from build123d import *

# Parameters (mm, degrees)
SKETCH2_W           = 100
SKETCH2_H           = 100
SKETCH2_R           = 12.5
BOSS_EXTRUDE1_DEPTH = 3
SKETCH3_W           = 7
SKETCH3_H           = 7
BOSS_EXTRUDE2_DEPTH = 5
SKETCH4_W           = 3
SKETCH4_H           = 8
SKETCH4_W_2         = 8
SKETCH4_H_2         = 3
BOSS_EXTRUDE3_DEPTH = 7
SKETCH5_R           = 1.6
CUT_EXTRUDE1_DEPTH  = 111.308657865
SKETCH8_R           = 1.6
CUT_EXTRUDE4_DEPTH  = 111.308657865
SKETCH9_R           = 3
CUT_EXTRUDE5_DEPTH  = 10
FILLET1_R           = 0.5


with BuildPart() as part:
    # Sketch2 → Boss-Extrude1 (new body)
    with BuildSketch(Plane(origin=(0, 0, 0), x_dir=(1, 0, 0), z_dir=(0, 1, 0))):
        Rectangle(SKETCH2_W, SKETCH2_H)
        with Locations(Location((0, 0, 0), (0, 0, 270))):
            Circle(SKETCH2_R, mode=Mode.SUBTRACT)
    extrude(amount=BOSS_EXTRUDE1_DEPTH)

    # Sketch3 → Boss-Extrude2 (add)
    with BuildSketch(Plane(origin=(0, 3, 0), x_dir=(1, 0, 0), z_dir=(0, 1, 0))):
        with Locations((-46.5, 46.5)):
            Rectangle(SKETCH3_W, SKETCH3_H)
        with Locations((46.5, 46.5)):
            Rectangle(SKETCH3_W, SKETCH3_H)
        with Locations((46.5, -46.5)):
            Rectangle(SKETCH3_W, SKETCH3_H)
        with Locations((-46.5, -46.5)):
            Rectangle(SKETCH3_W, SKETCH3_H)
    extrude(amount=BOSS_EXTRUDE2_DEPTH)

    # Sketch4 → Boss-Extrude3 (add)
    with BuildSketch(Plane.XZ):
        with Locations((46.5, -39)):
            Rectangle(SKETCH4_W, SKETCH4_H)
        with Locations((39, 46.5)):
            Rectangle(SKETCH4_W_2, SKETCH4_H_2)
        with Locations((-46.5, 39)):
            Rectangle(SKETCH4_W, SKETCH4_H)
        with Locations((-39, -46.5)):
            Rectangle(SKETCH4_W_2, SKETCH4_H_2)
    extrude(amount=BOSS_EXTRUDE3_DEPTH)

    # Sketch5 → Cut-Extrude1 (cut, through all)
    with BuildSketch(Plane(origin=(0, 0, -48), x_dir=(-1, 0, 0), z_dir=(0, 0, -1))):
        with Locations((39, -3.5)):
            Circle(SKETCH5_R)
        with Locations((-39, -3.5)):
            Circle(SKETCH5_R)
    extrude(amount=-CUT_EXTRUDE1_DEPTH, mode=Mode.SUBTRACT)

    # Sketch8 → Cut-Extrude4 (cut, through all)
    with BuildSketch(Plane(origin=(48, 0, 0), x_dir=(0, 0, -1), z_dir=(1, 0, 0))):
        with Locations((-39, -3.5)):
            Circle(SKETCH8_R)
        with Locations((39, -3.5)):
            Circle(SKETCH8_R)
    extrude(amount=-CUT_EXTRUDE4_DEPTH, mode=Mode.SUBTRACT)

    # Sketch9 → Cut-Extrude5 (cut)
    with BuildSketch(Plane(origin=(0, 3, 0), x_dir=(1, 0, 0), z_dir=(0, 1, 0))):
        with Locations(Location((-27.876571837, 0, 0), (0, 0, 270))):
            Circle(SKETCH9_R)
    extrude(amount=-CUT_EXTRUDE5_DEPTH, mode=Mode.SUBTRACT)

    # Fillet1
    fillet1_edges = [part.edges().sort_by_distance(p)[0] for p in [
        (-50, 4, 50),
        (-50, 4, -50),
        (50, 4, -50),
        (50, 4, 50),
    ]]
    fillet(fillet1_edges, radius=FILLET1_R)


solid = part.part
Work out the finished part from the listing and answer in its coordinate system (mm). A direction names the side the tool comes from. Give positions to 0.01 mm unless a question says otherwise; leave off trailing zeros. Write each loop counter-clockwise with the first axis right and the second up, starting at its lowest first coordinate (ties: lowest second). Pieces come first, ordered by that corner, then holes. Notation, with made-up numbers: (70, -26) - (90, -26) arc R20 ccw to (90, -20) - close; hole circle Ø4 at (-35, 61). An arc over 180 degrees is marked (long way). One line per item, written item: value. Start each with the question number.
1. For faces 1 (the flat face through (46, -3, -43)), 2 (the flat face through (43, 5, 47)), 3 (the flat face through (-43, -3, -47)), 4 (the flat face through (38, -2, 48)), 5 (the flat face through (-35, -3, -47)), determine the directions among +Z, -Z, +X, -X, +Y, -Y from which every point of the face is accessible in a straight line to the end or side of a thin tool.
2. Find section B-B (y = -3.5). State how many separate pieces and enclosed holes the cut face has, then the cut area to 3 significant figures.
3. Given pin 1 (2 mm diameter, centred on y = -4.5, z = 39.5, fed in from -X); pin 2 (3.5 mm diameter, centred on y = -5, z = 46.5, fed in from +X); pin 3 (0.9 mm diameter, centred on x = 47, y = -4, fed in from -Z); pin 4 (2 mm diameter, centred on y = 5, z = 19.5, fed in from -X), each flat-ended and moving along its own axis, determine where each tip first touches the part or whether it passes through.
4. Consider probe 1 along X at (y, z) = (0.7, 0); probe 2 along Y at (x, z) = (46.25, -39); probe 3 along Y at (x, z) = (-19.5, 21). Determine where each line is inside the solid, lowest interval first.
5. Find section A-A (z = 39). Write down the section's boundary in (x, y), then the cut area to 3 significant figures.
6. Find section D-D (z = 10). Write down the section's boundary in (x, y).
7. For a pull along Z with two mould halves and no side action, classify faces 6 (the flat face through (45, -2, -40)), 7 (the cylindrical face through (46.521, -1.914, -38.792)), 8 (the cylindrical face through (-30.805, 1.521, -0.65)), 9 (the flat face through (38, -2, 45)) as +Z half, -Z half, draft (parallel to the pull), parting line (faces both ways), or undercut.
8. Find section C-C (x = 39). Write down the section's boundary in (y, z), then the cut area to 3 significant figures.
Geometry results:
1. face 1: -Z, +X, -X, -Y
1. face 2: +Z, -Z, +Y
1. face 3: +Z, -Z, -X, -Y
1. face 4: +Z, +X, -X, -Y
1. face 5: +Z, -Z, +X, -Y
2. separate pieces: 8
2. enclosed holes: 0
2. area: 57.6 mm2
3. pin 1: x = -48
3. pin 2: x = 43
3. pin 3: z = -43
3. pin 4: through
4. probe 1: -50 to -30.88, -24.88 to -12.5, 12.5 to 50
4. probe 2: -7 to -5.1, -1.9 to 3
4. probe 3: 0 to 3
5. outline: (-50, 0) - (-48, 0) - (-48, -1.9) - (-45, -1.9) - (-45, 0) - (50, 0) - (50, 3) - (-50, 3) - close; (-48, -7) - (-45, -7) - (-45, -5.1) - (-48, -5.1) - close
5. area: 311 mm2
6. outline: (-50, 0) - (-7.5, 0) - (-7.5, 3) - (-50, 3) - close; (7.5, 0) - (50, 0) - (50, 3) - (7.5, 3) - close
7. face 6: draft
7. face 7: undercut
7. face 8: undercut
7. face 9: -Z half
8. outline: (-7, 45) - (-5.1, 45) - (-5.1, 48) - (-7, 48) - close; (-1.9, 45) - (0, 45) - (0, -50) - (3, -50) - (3, 50) - (0, 50) - (0, 48) - (-1.9, 48) - close
8. area: 311 mm2
